Source: CAD feature listing. Evaluate the final solid. Frame: model axes, mm. Face numbers are marked on the shaded views. A direction names the side the tool comes from. Round coordinates to 2 decimals unless told otherwise and drop trailing zeros. Write each loop counter-clockwise with the first axis right and the second up, starting at its lowest first coordinate (ties: lowest second). Pieces come first, ordered by that corner, then holes.
```python
from build123d import *

# Parameters (mm, degrees)
F0_R     = 31.75
F0_R_2   = 3.175
F0_R_3   = 15.875
F1_DEPTH = 6.35
F0_R_4   = 9.525
F2_DEPTH = 19.05


with BuildPart() as f1:
    # F0 (on Top) → F1 (new body, symmetric)
    with BuildSketch(Plane.XY):
        Circle(F0_R)
        with Locations((0, -25.4)):
            Circle(F0_R_2, mode=Mode.SUBTRACT)
        with Locations((-25.4, 0)):
            Circle(F0_R_2, mode=Mode.SUBTRACT)
        Circle(F0_R_3, mode=Mode.SUBTRACT)
        with Locations((25.4, 0)):
            Circle(F0_R_2, mode=Mode.SUBTRACT)
        with Locations((0, 25.4)):
            Circle(F0_R_2, mode=Mode.SUBTRACT)
    extrude(amount=F1_DEPTH, both=True)

    # F0 (on Top) → F2 (join)
    with BuildSketch(Plane.XY):
        Circle(F0_R_3)
        Circle(F0_R_4, mode=Mode.SUBTRACT)
    extrude(amount=F2_DEPTH)


solid = f1.part
```
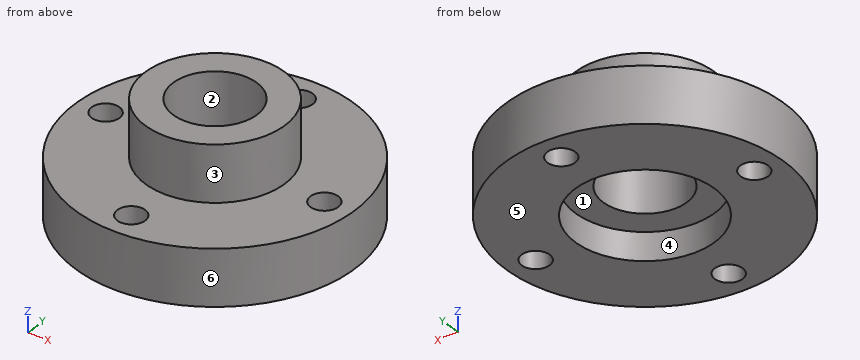
Q1. Line query: line 1 (Y direction, x = 0, z = 0.5) (3 decimals); line 2 (Y direction, x = 0, z = -3.5) (3 decimals); line 3 (Z direction, x = 17, y = 20). Output: solid intervals per line, ascending.
Q2. Set-up query: the marked faces 1, 2 and 3. Return all of +Z, -Z, +X, -X, +Y, -Y with unobstructed straight access to the full face (end or side cutting, diameter ignored); none if empty.
Q3. Pin query (flat end, axial travel): P1, Ø5, axis at x = -25.4, y = 0, coming from the -Z side; P2, Ø1.5, axis at x = 12.5, z = 10, coming from the -Y side; P3, Ø16, axis at x = -3, y = -1.5, coming from the -Z side; P4, Ø12, axis at x = 24, y = -19.5, coming from the +Z side. Return the tip coordinate at first contact, or that it passes through.
Q4. Section query A-A, the plane y = -25.4. Output: boundary loops of the cut face in (x, z) (3 decimals).
Q5. Mould query, pull axis X, two halves, no side actions, for the marked faces 4, 5 and 6. Classes: pulls with the +X half, pulls with the -X half, needs draft (parallel to the pull), parting line crosses it, or undercut.
Q6. Section query C-C, the plane y = 0. Output: boundary loops of the cut face in (x, z) (3 decimals).
Filled in:
1. line 1: y = -31.75 to -28.575, -22.225 to -9.525, 9.525 to 22.225, 28.575 to 31.75
1. line 2: y = -31.75 to -28.575, -22.225 to -15.875, 15.875 to 22.225, 28.575 to 31.75
1. line 3: z = -6.35 to 6.35
2. face 1: -Z
2. face 2: +Z, -Z
2. face 3: +Z
3. P1: passes through
3. P2: stops at y = -10.67
3. P3: stops at z = 0
3. P4: stops at z = 6.35
4. outline: (-19.05, -6.35) - (-3.175, -6.35) - (-3.175, 6.35) - (-19.05, 6.35) - close; (3.175, -6.35) - (19.05, -6.35) - (19.05, 6.35) - (3.175, 6.35) - close
5. face 4: undercut
5. face 5: needs draft
5. face 6: parting line crosses it
6. outline: (-31.75, -6.35) - (-28.575, -6.35) - (-28.575, 6.35) - (-31.75, 6.35) - close; (-22.225, -6.35) - (-15.875, -6.35) - (-15.875, 0) - (-9.525, 0) - (-9.525, 19.05) - (-15.875, 19.05) - (-15.875, 6.35) - (-22.225, 6.35) - close; (9.525, 0) - (15.875, 0) - (15.875, -6.35) - (22.225, -6.35) - (22.225, 6.35) - (15.875, 6.35) - (15.875, 19.05) - (9.525, 19.05) - close; (28.575, -6.35) - (31.75, -6.35) - (31.75, 6.35) - (28.575, 6.35) - close
